Source: CAD feature listing. Evaluate the final solid. Frame: model axes, mm. A direction names the side the tool comes from. Coordinates: 2 decimals unless noted, no trailing zeros. Write each loop counter-clockwise with the first axis right and the second up, starting at its lowest first coordinate (ties: lowest second). Pieces come first, ordered by that corner, then holes. Notation, with made-up numbers: (2.5, -21.5) - (57.5, -21.5) arc R12 ccw to (57.5, -5.5) - close; hole circle Ø2 at (-12, 68). An arc over 180 degrees is marked (long way). One line per question, with ' | ' between items.
from build123d import *

# Parameters (mm, degrees)
SKETCH_1_W          = 70
SKETCH_1_H          = 50
EXTRUDE_1_DEPTH     = 3
EXTRUDE_2_DEPTH     = 70
SKETCH_3_R          = 1.6
EXTRUDE_3_DEPTH     = 3
EXTRUDE_4_REACH     = 139.875
SKETCH_4_W          = 70
SKETCH_4_H          = 5.267949192
FILLET_1_R          = 5
SKETCH_5_W          = 70
SKETCH_5_H          = 28.866025404
CUT_EXTRUDE_1_DEPTH = 138.47436204
SKETCH_6_W          = 70
SKETCH_6_H          = 3
CUT_EXTRUDE_2_DEPTH = 133.365261865
FILLET_2_R          = 5


with BuildPart() as part:
    # 草图1 → 凸台-拉伸1 (new body)
    with BuildSketch(Plane(origin=(0, 0, 0), x_dir=(1, 0, 0), z_dir=(0, 1, 0))):
        with Locations((35, 25)):
            Rectangle(SKETCH_1_W, SKETCH_1_H)
    extrude(amount=EXTRUDE_1_DEPTH)

    # 草图2 → 凸台-拉伸2 (add)
    with BuildSketch(Plane.ZY):
        Polygon((0, 15), (-6.062177826, 18.5), (-4.562177826, 21.098076211), (4, 16.154700538), (4, 15), (4, 0), (0, 0), align=None)
    extrude(amount=-EXTRUDE_2_DEPTH)

    # 草图3 → 凸台-拉伸3 (add)
    with BuildSketch(Plane(origin=(0, 13.848076211, 7.995190528), x_dir=(1, 0, 0), z_dir=(0, 0.86602540378444, 0.49999999999999784))):
        with BuildLine():
            Line((-48.265, 11.613248654), (-36.265, 11.613248654))
            Line((-36.265, 11.613248654), (106.265, 11.613248654))
            Line((106.265, 11.613248654), (118.265, 11.613248654))
            ThreePointArc((118.265, 11.613248654), (125.265, 4.613248654), (118.265, -2.386751346))
            Line((118.265, -2.386751346), (106.265, -2.386751346))
            Line((106.265, -2.386751346), (-36.265, -2.386751346))
            Line((-36.265, -2.386751346), (-48.265, -2.386751346))
            ThreePointArc((-48.265, -2.386751346), (-55.265, 4.613248654), (-48.265, 11.613248654))
        make_face()
        with Locations(Location((-36.265, 4.613248654, 0), (0, 0, 270))):
            Circle(SKETCH_3_R, mode=Mode.SUBTRACT)
        with Locations(Location((106.265, 4.613248654, 0), (0, 0, 270))):
            Circle(SKETCH_3_R, mode=Mode.SUBTRACT)
        with Locations(Location((-48.265, 4.613248654, 0), (0, 0, 270))):
            Circle(SKETCH_3_R, mode=Mode.SUBTRACT)
        with Locations(Location((118.265, 4.613248654, 0), (0, 0, 270))):
            Circle(SKETCH_3_R, mode=Mode.SUBTRACT)
    extrude(amount=-EXTRUDE_3_DEPTH)

    # 凸台-拉伸4: up to this face of the body (flat: up to its plane)
    extrude_4_end = Plane(part.part.faces().sort_by_distance((35, 6.345299462, 4))[0])
    # 草图4 → 凸台-拉伸4 (add, up to the picked face)
    with BuildSketch(Plane(origin=(0, 11.25, 6.495190528), x_dir=(1, 0, 0), z_dir=(0, -0.8660254037844396, -0.4999999999999982)), mode=Mode.PRIVATE) as extrude_4_sk1:
        with Locations((35, -0.24722325)):
            Rectangle(SKETCH_4_W, SKETCH_4_H)
    extrude_4_tool1 = split(extrude(extrude_4_sk1.sketch, amount=EXTRUDE_4_REACH, mode=Mode.PRIVATE), bisect_by=extrude_4_end, keep=Keep.BOTH, mode=Mode.PRIVATE)
    add(extrude_4_tool1.solids().sort_by(Axis((35, 11.373612, 6.281089), (0, -0.8660254037844396, -0.4999999999999982)))[0])

    # 圆角1
    fillet_1_edges = [part.edges().sort_by_distance(p)[0] for p in [
        (35, 3, 0),
    ]]
    fillet(fillet_1_edges, radius=FILLET_1_R)

    # 草图5 → 切除-拉伸1 (cut, through all)
    with BuildSketch(Plane(origin=(0, -1.193375673, 2.066987298), x_dir=(1, 0, 0), z_dir=(-1.4881366732147052e-15, -0.49999999999999784, 0.8660254037844398))):
        with Locations((35, -10.566987298)):
            Rectangle(SKETCH_5_W, SKETCH_5_H)
    extrude(amount=CUT_EXTRUDE_1_DEPTH, mode=Mode.SUBTRACT)

    # 草图6 → 切除-拉伸2 (cut, through all)
    with BuildSketch(Plane(origin=(0, 5.806624327, -10.057368355), x_dir=(-1, 0, 0), z_dir=(0, 0.49999999999999784, -0.8660254037844398))):
        with Locations((-35, 14.490381057)):
            Rectangle(SKETCH_6_W, SKETCH_6_H)
    extrude(amount=CUT_EXTRUDE_2_DEPTH, mode=Mode.SUBTRACT)

    # 圆角2
    fillet_2_edges = [part.edges().sort_by_distance(p)[0] for p in [
        (0, 1.5, -50),
        (70, 1.5, -50),
    ]]
    fillet(fillet_2_edges, radius=FILLET_2_R)


solid = part.part
Item 1: Pin query (flat end, axial travel): pin 1 Ø3 at (x, y) = (7.5, 11) entering from +Z; pin 2 Ø2 at (x, y) = (37.5, 11) entering from -Z; pin 3 Ø4.5 at (y, z) = (5, -27) entering from +X. Return the tip coordinate at first contact, or that it passes through.
Check sheet entries:
pin 1: z = 9.97 | pin 2: z = 0 | pin 3: x = 70
Item 2: Mould query, pull axis Z, two halves, no side actions, for faces 4 (the face through (-55.263, 14.797, 3.394)), 5 (the face through (1, 2, -48)), 6 (the face through (-46.92, 14.44, 4.01)), 7 (the face through (33.83, 7.82, 7.27)). Classes: pulls with the +Z half, pulls with the -Z half, needs draft (parallel to the pull), parting line crosses it, or undercut.
Check sheet entries:
face 4: parting line crosses it | face 5: pulls with the -Z half | face 6: undercut | face 7: pulls with the +Z half
Item 3: Ray query, line 1 along Y through (x, z) = (42.5, -19.5); line 2 along X through (y, z) = (5, 1.5); line 3 along Z through (x, y) = (80, 16.75). Return the intervals inside material, ascending. Write a range as [from, to].
Check sheet entries:
line 1: [0, 3] | line 2: [0, 70] | line 3: [-3.03, 2.97]
Item 4: Cut plane A-A on x = 14.5. Return loops of the section in (y, z), and give its area (3 significant figures).
Check sheet entries:
outline: (0, -50) - (3, -50) - (3, -5) arc R5 cw to (8, 0) - (15, 0) - (17.06, -3.56) - (19.65, -2.06) - (12.65, 10.06) - (0, 2.76) - close | area: 275 mm²
Item 5: Cut plane C-C on x = 86. Return loops of the section in (y, z).
Check sheet entries:
outline: (10.06, 8.56) - (17.06, -3.56) - (19.65, -2.06) - (12.65, 10.06) - close
Item 6: Cut plane B-B on z = -37. Return loops of the section in (x, y).
Check sheet entries:
outline: (0, 0) - (70, 0) - (70, 3) - (0, 3) - close
Item 7: Access query for faces 1 (the face through (35, 3, -28)), 2 (the face through (-34.92, 14.44, 4.01)), 3 (the face through (35, 4, -2)). Directions: +Z, -Z, +X, -X, +Y, -Y. A direction counts if a zero-diameter tool reaches every point of the face in a straight line with its end or side. Return the directions, or none.
Check sheet entries:
face 1: -Z, +X, -X, +Y | face 2: none | face 3: -Z, +X, -X
